Autodesk Inventor part; units mm, degrees
ref_plane "YZ Plane" through (0, 0, 0) normal (1, 0, 0) x (0, 1, 0)
ref_plane "XZ Plane" through (0, 0, 0) normal (0, 1, 0) x (-1, 0, 0)
ref_plane "XY Plane" through (0, 0, 0) normal (0, 0, 1) x (1, 0, 0)
sketch "Sketch1" plane through (0, 0, 0) normal (0, 0, 1) x (1, 0, 0)
  line L0 (12.7, -25.4) -> (-12.7, -25.4)
  line L1 (-12.7, -25.4) -> (-12.7, 25.4)
  line L2 (-12.7, 25.4) -> (12.7, 25.4)
  line L3 (12.7, 25.4) -> (12.7, -25.4)
  line L4 (12.7, -25.4) -> (-12.7, 25.4) construction
  line L5 (-12.7, -25.4) -> (12.7, 25.4) construction
  line L6 (10.16, -22.86) -> (-10.16, -22.86)
  line L7 (-10.16, -22.86) -> (-10.16, 22.86)
  line L8 (-10.16, 22.86) -> (10.16, 22.86)
  line L9 (10.16, 22.86) -> (10.16, -22.86)
  line L10 (10.16, -22.86) -> (-10.16, 22.86) construction
  line L11 (-10.16, -22.86) -> (10.16, 22.86) construction
  point P0 (0, 0)
  dimension "d0" = 25.4
  dimension "d1" = 50.8
  dimension "d2" = 20.32
  dimension "d3" = 45.72
extrude "Extrusion1" add sketch "Sketch1" along normal mid plane 127
sketch "Sketch2" plane through (-12.7, 25.4, 63.5) normal (0, 1, 0) x (1, 0, 0)
  line L0 (0, 0) -> (0, 127)
  line L1 (25.4, 0) -> (0, 0)
  point P0 (12.7, 63.5)
  point P1 (12.7, 12.7)
  dimension "d6" = 12.7
  dimension "d7" = 12.7
hole "Hole1" at (0, 25.4, 50.8) direction (0, -1, 0) diameter 4.1402 end through all
pattern_linear "Rectangular Pattern1" count 5 spacing 25.4 along (0, 0, -1) of "Hole1"
properties part number "Elevator_stationary_extender"
Can you work these out from the model? Positions are in its coordinate system, mm. A direction names the side the tool comes from. Round coordinates to 2 decimals unless told otherwise and drop trailing zeros. Loops run counter-clockwise (first coordinate to the right, second up) from the corner with the lowest first, then second, coordinate; pieces in that order, holes last. Notation, with made-up numbers: (61.5, 48) -> (84.5, 48) arc R12 ccw to (84.5, 58) -> close; hole circle Ø4 at (66, 82.5). An arc over 180 degrees is marked (long way). Answer in a Markdown table with one row per item.
Item 1: Suppose I cut it at D-D, the plane z = 47.5. List the corners of the cut face in (x, y) for me, plus the area to 3 significant figures.
Answer block:
| item | result |
|---|---|
| outline | (-12.7, -25.4) -> (12.7, -25.4) -> (12.7, 25.4) -> (-12.7, 25.4) -> close; hole (-10.16, -22.86) -> (10.16, -22.86) -> (10.16, 22.86) -> (-10.16, 22.86) -> close |
| area | 361 mm² |
Item 2: We'd pull the mould along X, two halves only. Please class faces 1 (the flat face through (-10.4, 2, -63.5)), 2 (the flat face through (10.16, 0, -1)), 3 (the flat face through (12.7, 0, -1)): released by +X, released by -X, zero draft, split by the parting line, or undercut.
Answer block:
| item | result |
|---|---|
| face 1 | zero draft |
| face 2 | undercut |
| face 3 | released by +X |
Item 3: Suppose I cut it at C-C, the plane x = -3.25. List the corners of the cut face in (y, z) for me.
Answer block:
| item | result |
|---|---|
| outline | (-25.4, -63.5) -> (-22.86, -63.5) -> (-22.86, 63.5) -> (-25.4, 63.5) -> close; (22.86, -63.5) -> (25.4, -63.5) -> (25.4, 63.5) -> (22.86, 63.5) -> close |
Item 4: Will this pin go through, and if not, where does the flat tip stop? P1, Ø3.5, axis at x = 0, z = -50.8, coming from the -Y side.
Answer block:
| item | result |
|---|---|
| P1 | through |
Item 5: Suppose I cut it at A-A, the plane z = -50.8. List the corners of the cut face in (x, y) for me, plus the area to 3 significant figures.
Answer block:
| item | result |
|---|---|
| outline | (-12.7, -25.4) -> (-2.07, -25.4) -> (-2.07, -22.86) -> (-10.16, -22.86) -> (-10.16, 22.86) -> (-2.07, 22.86) -> (-2.07, 25.4) -> (-12.7, 25.4) -> close; (2.07, -25.4) -> (12.7, -25.4) -> (12.7, 25.4) -> (2.07, 25.4) -> (2.07, 22.86) -> (10.16, 22.86) -> (10.16, -22.86) -> (2.07, -22.86) -> close |
| area | 340 mm² |
Item 6: Suppose I cut it at B-B, the plane y = -12.5. List the corners of the cut face in (x, z) for me, plus the area to 3 significant figures.
Answer block:
| item | result |
|---|---|
| outline | (-12.7, -63.5) -> (-10.16, -63.5) -> (-10.16, 63.5) -> (-12.7, 63.5) -> close; (10.16, -63.5) -> (12.7, -63.5) -> (12.7, 63.5) -> (10.16, 63.5) -> close |
| area | 645 mm² |
Item 7: On a 3-axis mill with a long thin cutter (end or side, diameter ignored), from which of +Z, -Z, +X, -X, +Y, -Y can I reach the whole of each face in a straight line? I mean faces 4 (the flat face through (-10.16, 0, -1)), 5 (the flat face through (-3, -25.4, -1)). Say none if no direction works.
Answer block:
| item | result |
|---|---|
| face 4 | +Z, -Z |
| face 5 | +Z, -Z, +X, -X, -Y |
Item 8: If I drill on probe 1 along Z at (x, y) = (0, 23.6); probe 2 along Y at (x, z) = (4.5, -33); probe 3 along X at (y, z) = (-11.5, 41), over which ranges is the centre line in solid material (lowest first)?
Answer block:
| item | result |
|---|---|
| probe 1 | -63.5 to -52.87, -48.73 to -27.47, -23.33 to -2.07, 2.07 to 23.33, 27.47 to 48.73, 52.87 to 63.5 |
| probe 2 | -25.4 to -22.86, 22.86 to 25.4 |
| probe 3 | -12.7 to -10.16, 10.16 to 12.7 |
